The figure shows three views and two pictorial views of one solid part (mm, origin at its lowest corner). Answer the questions. Round coordinates to 2 decimals unless told otherwise and drop trailing zeros. Order: outer loops, then holes, each group sorted by start corner. A loop starts at its lowest first (then second) coordinate and runs counter-clockwise, first axis right, second up. Notation, with made-up numbers: (-10, 76) -> (23, 76) arc R19 cw to (23, 88) -> close; hole circle Ø11 at (87.25, 1.25). An arc over 180 degrees is marked (long way). Return JSON: item names as keys, results as strings. Group by question number.
(1) The part is cut by section A-A (z = 73). Determine the outline of the cut face in (x, y).
(2) Consider line 1 (X direction, y = 1, z = 73); line 2 (Z direction, x = 66.5, y = 1.25); line 3 (X direction, y = 3.55, z = 10.5). Determine where each line is inside the solid, lowest interval first. Write a range as [from, to].
(3) Each of these flat-tipped pins is pushed along its axis until it touches: pin 1 (3 mm diameter, centred on x = 7.5, y = 10.5, fed in from +Z); pin 2 (7.5 mm diameter, centred on x = 8, y = 9.5, fed in from -Z); pin 3 (6 mm diameter, centred on x = 71.5, z = 11, fed in from +Y). Where does it stop, or does it pass through?
(4) Determine the mould class of the marked faces 1 and 2 for opening direction X: +X half, -X half, draft (parallel to the pull), parting line (faces both ways), or undercut.
(5) The part is cut by section B-B (x = 28). Determine the outline of the cut face in (y, z).
(6) The part is cut by section C-C (z = 45). Determine the outline of the cut face in (x, y), plus the area to 3 significant figures.
(7) The part is cut by section D-D (x = 127). Determine the outline of the cut face in (y, z), plus the area to 3 significant figures.
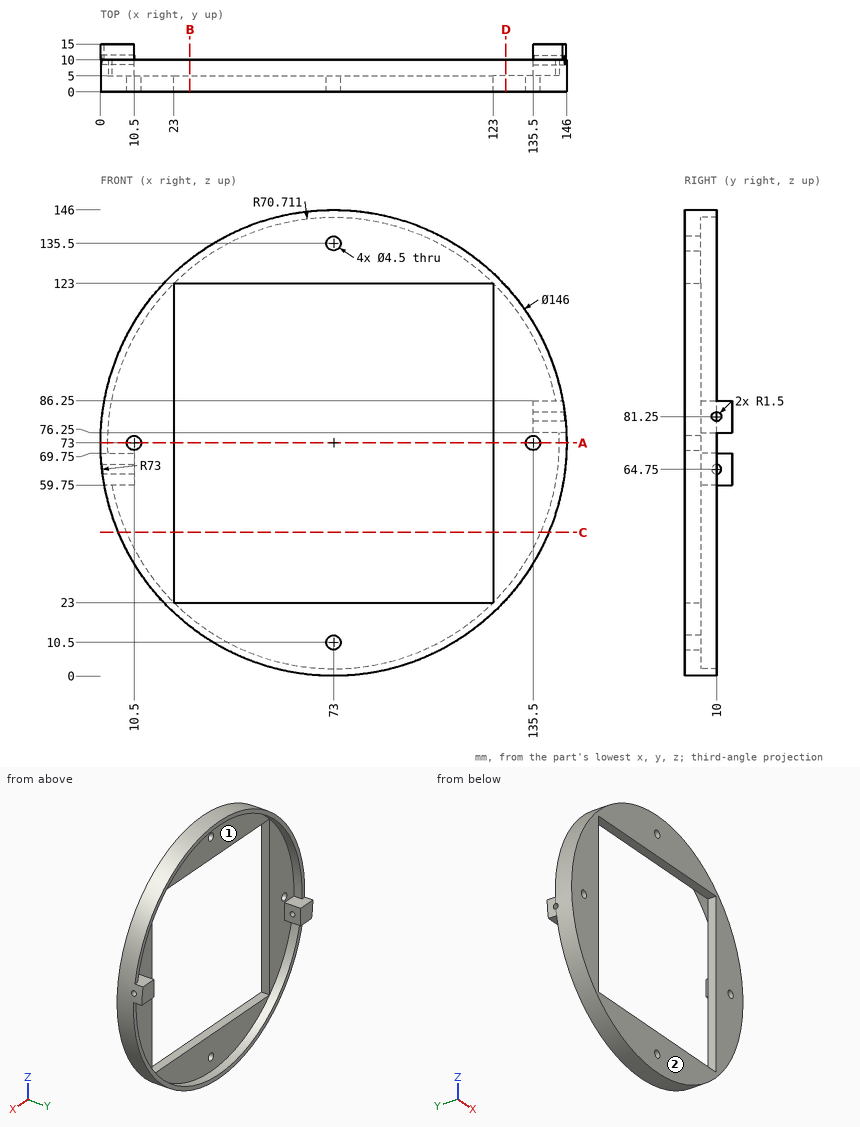
Answer below:
{
 "1": {"outline": "(0, 0) -> (8.25, 0) -> (8.25, 5) -> (2.29, 5) -> (2.29, 10) -> (0, 10) -> close; (12.75, 0) -> (23, 0) -> (23, 5) -> (12.75, 5) -> close; (123, 0) -> (133.25, 0) -> (133.25, 5) -> (123, 5) -> close; (137.75, 0) -> (146, 0) -> (146, 10) -> (143.71, 10) -> (143.71, 5) -> (137.75, 5) -> close"},
 "2": {"line 1": "x = [0, 8.25], [12.75, 23], [123, 133.25], [137.75, 146]", "line 2": "z = [0.29, 23], [123, 145.71]", "line 3": "x = [35.28, 70.75], [75.25, 110.72]"},
 "3": {"pin 1": "stops at z = 107.96", "pin 2": "stops at z = 33.28", "pin 3": "stops at y = 5"},
 "4": {"face 1": "undercut", "face 2": "draft"},
 "5": {"outline": "(0, 15.52) -> (10, 15.52) -> (10, 18.46) -> (5, 18.46) -> (5, 23) -> (0, 23) -> close; (0, 123) -> (5, 123) -> (5, 127.54) -> (10, 127.54) -> (10, 130.48) -> (0, 130.48) -> close"},
 "6": {"outline": "(5.58, 0) -> (23, 0) -> (23, 5) -> (8.07, 5) -> (8.07, 10) -> (5.58, 10) -> close; (123, 0) -> (140.42, 0) -> (140.42, 10) -> (137.93, 10) -> (137.93, 5) -> (123, 5) -> close", "area": "199 mm²"},
 "7": {"outline": "(0, 23.88) -> (10, 23.88) -> (10, 27.35) -> (5, 27.35) -> (5, 118.65) -> (10, 118.65) -> (10, 122.12) -> (0, 122.12) -> close", "area": "526 mm²"}
}
